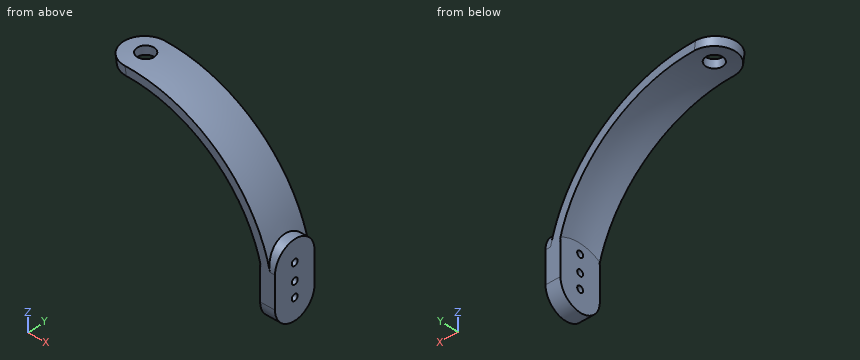
```python
from build123d import *

# Parameters (mm, degrees)
REVOLVE_1_ANGLE           = 98.68117871
REVOLVE_1_OTHER_WAY_ANGLE = 8.68117871
SKETCH_3_R                = 4
CUT_EXTRUDE_1_DEPTH       = 100.498743711
SKETCH_4_R                = 1.5
CUT_EXTRUDE_2_DEPTH       = 100.41830825
CUT_EXTRUDE_3_DEPTH       = 102.960221512
FILLET_1_R                = 10
EXTRUDE_START             = -7
SKETCH_8_R                = 1.5
EXTRUDE_1_DEPTH           = 7


with BuildPart() as part:
    # 草图2 → 旋转1 (revolve)
    with BuildSketch(Plane.XY):
        with BuildLine():
            Line((65.238025721, 10), (69.282032303, 10))
            ThreePointArc((69.282032303, 10), (70, 0), (69.282032303, -10))
            Line((69.282032303, -10), (65.238025721, -10))
            ThreePointArc((65.238025721, -10), (66, 0), (65.238025721, 10))
        make_face()
    revolve(axis=Axis((0, 0, 0), (0, -1, 0)), revolution_arc=REVOLVE_1_ANGLE)

    # 草图2 → 旋转1 other way (revolve)
    with BuildSketch(Plane.XY):
        with BuildLine():
            Line((65.238025721, 10), (69.282032303, 10))
            ThreePointArc((69.282032303, 10), (70, 0), (69.282032303, -10))
            Line((69.282032303, -10), (65.238025721, -10))
            ThreePointArc((65.238025721, -10), (66, 0), (65.238025721, 10))
        make_face()
    revolve(axis=Axis((0, 0, 0), (0, 1, 0)), revolution_arc=REVOLVE_1_OTHER_WAY_ANGLE)

    # 草图3 → 切除-拉伸1 (cut, through all)
    with BuildSketch(Plane.XY):
        with Locations(Location((0, 0, 0), (0, 0, 180))):
            Circle(SKETCH_3_R)
    extrude(amount=CUT_EXTRUDE_1_DEPTH, mode=Mode.SUBTRACT)

    # 草图4 → 切除-拉伸2 (cut, through all)
    with BuildSketch(Plane(origin=(0, 0, 0), x_dir=(0, 0, -1), z_dir=(1, 0, 0))):
        with Locations(Location((0, 0, 0), (0, 0, 180))):
            Circle(SKETCH_4_R)
    extrude(amount=CUT_EXTRUDE_2_DEPTH, mode=Mode.SUBTRACT)

    # 草图7 → 切除-拉伸3 (cut, through all)
    with BuildSketch(Plane(origin=(63, 0, 0), x_dir=(0, 0, -1), z_dir=(1, 0, 0))):
        with BuildLine():
            Line((25, -10), (-15, -10))
            ThreePointArc((-15, -10), (-25, 0), (-15, 10))
            Line((-15, 10), (25, 10))
            Line((25, 10), (25, -10))
        make_face()
    extrude(amount=CUT_EXTRUDE_3_DEPTH, mode=Mode.SUBTRACT)

    # 圆角1
    # the kernel refuses this fillet: 10 mm, written as the material it takes off along each edge
    with BuildSketch(Plane(origin=(-6.073370605, 10, 39.777039651), x_dir=(0.9885435216678339, 0, 0.15093609829512958), z_dir=(-0.15093609829512958, 0, 0.9885435216678339)), Plane(origin=(-14.230562095, -10, 93.201892243), x_dir=(0.9885435216678339, 0, 0.15093609829512958), z_dir=(0.15093609829512958, 0, -0.9885435216678339))) as fillet_1_piece_1:
        with BuildLine():
            CenterArc((FILLET_1_R, -FILLET_1_R), FILLET_1_R, 90, 90)
            Line((0, -FILLET_1_R), (0, 0))
            Line((0, 0), (FILLET_1_R, 0))
        make_face()
    extrude(amount=54.044006582, mode=Mode.SUBTRACT)

    # 草图8 → 凸台-拉伸1 (add)
    with BuildSketch(Plane(origin=(70, 0, 0), x_dir=(0, 0, -1), z_dir=(1, 0, 0)).offset(EXTRUDE_START)):
        with BuildLine():
            Line((-15, 10), (0, 10))
            ThreePointArc((0, 10), (10, 0), (0, -10))
            Line((0, -10), (-15, -10))
            ThreePointArc((-15, -10), (-25, 0), (-15, 10))
        make_face()
        Circle(SKETCH_8_R, mode=Mode.SUBTRACT)
        with Locations((-7, 0)):
            Circle(SKETCH_8_R, mode=Mode.SUBTRACT)
        with Locations((-15, 0)):
            Circle(SKETCH_8_R, mode=Mode.SUBTRACT)
    extrude(amount=EXTRUDE_1_DEPTH)


solid = part.part
```
Input: part model. Units: mm. Frame: model coordinates. Round coordinates to 2 decimals unless told otherwise and drop trailing zeros. Loops run counter-clockwise (first coordinate to the right, second up) from the corner with the lowest first, then second, coordinate; pieces in that order, holes last. Notation, with made-up numbers: (-17, -16) -> (25, -16) arc R9 ccw to (25, -5) -> close; hole circle Ø2 at (-18, -7.5). An arc over 180 degrees is marked (long way). Use one line per item in the form item = value. Start each with the question number.
Item 1: Section query C-C on y = 0. Return the cut outline in (x, z).
Item 2: Section query D-D on z = 23. Return the cut outline in (x, y), then the cut area to 3 significant figures.
Item 3: Section query A-A on z = 7. Return the cut outline in (x, y), then the cut area to 3 significant figures.
Item 4: Section query B-B on y = -7. Return the cut outline in (x, z).
Item 5: Contact query for flat-ended pins moving along their axis: pin 1 Ø3.5 at (y, z) = (0, 7) entering from -X; pin 2 Ø1.5 at (x, y) = (16, -0.5) entering from +Z; pin 3 Ø1.5 at (x, y) = (39, -7) entering from -Z. Output: stop coordinate, or through.
Item 6: Material intervals for L1, parallel to Y at x = 0, z = 68.4; L2, parallel to Y at x = 67, z = 7; L3, parallel to X at y = -1.25, z = 13, sorted ascending. Write a range as from..to.
Ans:
q1.outline = (-10.57, 69.2) -> (-9.96, 65.24) arc R66 cw to (-4, 65.88) -> (-4, 69.89) arc R70 ccw to start; (4, 65.88) arc R66 cw to (63, 19.67) -> (63, 16.5) -> (70, 16.5) -> (70, 25) -> (65.38, 25) arc R70 ccw to (4, 69.89) -> close; (63, -10) -> (70, -10) -> (70, -1.5) -> (63, -1.5) -> close; (63, 1.5) -> (70, 1.5) -> (70, 5.5) -> (63, 5.5) -> close; (63, 8.5) -> (70, 8.5) -> (70, 13.5) -> (63, 13.5) -> close
q2.outline = (61.05, -10) -> (65.35, -10) arc R66.11 ccw to (65.84, -6) -> (70, -6) -> (70, 6) -> (65.84, 6) arc R66.11 ccw to (65.35, 10) -> (61.05, 10) arc R61.86 cw to start
q2.area = 133 mm^2
q3.outline = (63, -10) -> (70, -10) -> (70, -1.5) -> (63, -1.5) -> close; (63, 1.5) -> (70, 1.5) -> (70, 10) -> (63, 10) -> close
q3.area = 119 mm^2
q4.outline = (-7.68, 69.22) -> (-7.07, 65.25) arc R65.63 cw to (63, 18.38) -> (63, -7.14) -> (70, -7.14) -> (70, 22.14) -> (66.04, 22.14) arc R69.65 ccw to start
q5.pin_1 = 63
q5.pin_2 = 68.32
q5.pin_3 = 52.21
q6.L1 = -10..-4, 4..10
q6.L2 = -10..-1.5, 1.5..10
q6.L3 = 63..70
